Design review of the part built by this model. Coordinates are the model's own, in mm. A direction names the side the tool comes from. Round coordinates to 2 decimals unless told otherwise and drop trailing zeros. Loops run counter-clockwise (first coordinate to the right, second up) from the corner with the lowest first, then second, coordinate; pieces in that order, holes last. Notation, with made-up numbers: (-15.75, 32.25) - (4.25, 32.25) arc R32 ccw to (4.25, 59.25) - close; hole circle Ø3 at (3, 58). An arc over 180 degrees is marked (long way). Use one line per item in the form item = value. Start each with the question number.
(1) Wall thickness on probe 1 along X at (y, z) = (-131, -670); probe 2 along Y at (x, z) = (157, -182); probe 3 along X at (y, z) = (17.5, -85): over which ranges is each line inside the solid? List them lowest first. Write a range as [from, to].
(2) For pin 1 (4 mm diameter, centred on y = -19, z = -359.5, fed in from +X); pin 2 (1.5 mm diameter, centred on x = 870, z = -256, fed in from -Y), all flat-tipped, find the tip position at first contact; note any pin that passes through.
(3) We need section A-A, the plane y = -92. Write out the cut boundary in (x, z).
(4) We need section C-C, the plane y = 26. Write out the cut boundary in (x, z), then the cut area to 3 significant figures.
(5) Machinability: for faces 1 (the cylindrical face through (277.636, 20.28, -249.322)), 2 (the flat face through (913, 11, 0)), 3 (the flat face through (492, 0, -608)), which of the approach directions +Z, -Z, +X, -X, +Y, -Y give a long, thin tool a straight path to every point of the face, cutting with its end or side? Answer none if there is none.
(6) We need section D-D, the plane x = 549. Write out the cut boundary in (y, z), then the cut area to 3 significant figures.
(7) We need section B-B, the plane z = -532. Write out the cut boundary in (x, y).
from build123d import *

# Parameters (mm, degrees)
SKETCH1_W           = 1000
SKETCH1_H           = 1200
BOSS_EXTRUDE1_DEPTH = 40
SKETCH2_W           = 44.100266395
SKETCH2_H           = 1200
SKETCH2_W_2         = 40
BOSS_EXTRUDE2_DEPTH = 140
FILLET1_R           = 70
SKETCH3_R           = 334.802588384
CUT_EXTRUDE2_DEPTH  = 140


with BuildPart() as part:
    # Sketch1 → Boss-Extrude1 (new body)
    with BuildSketch(Plane(origin=(0, 0, 0), x_dir=(1, 0, 0), z_dir=(0, 1, 0))):
        with Locations((500, 600)):
            Rectangle(SKETCH1_W, SKETCH1_H)
    extrude(amount=BOSS_EXTRUDE1_DEPTH)

    # Sketch2 → Boss-Extrude2 (add)
    with BuildSketch(Plane.XZ):
        with Locations((977.949866803, -600)):
            Rectangle(SKETCH2_W, SKETCH2_H)
        with Locations((20, -600)):
            Rectangle(SKETCH2_W_2, SKETCH2_H)
    extrude(amount=BOSS_EXTRUDE2_DEPTH)

    # Fillet1
    fillet1_edges = [part.edges().sort_by_distance(p)[0] for p in [
        (1000, 40, -600),
        (0, 40, -600),
    ]]
    fillet(fillet1_edges, radius=FILLET1_R)

    # Sketch3 → Cut-Extrude2 (cut)
    with BuildSketch(Plane(origin=(0, 40, 0), x_dir=(1, 0, 0), z_dir=(0, 1, 0))):
        with Locations((500, 1200)):
            Circle(SKETCH3_R)
        with BuildLine():
            Line((221.441080201, 0), (780, 0))
            ThreePointArc((780, 0), (725.321357402, 246.103392604), (571.573934725, 445.899197935))
            ThreePointArc((571.573934725, 445.899197935), (500.7205401, 471.613897531), (429.867145476, 445.899197935))
            ThreePointArc((429.867145476, 445.899197935), (276.119722799, 246.103392604), (221.441080201, 0))
        make_face()
    extrude(amount=-CUT_EXTRUDE2_DEPTH, mode=Mode.SUBTRACT)


solid = part.part
Data:
q1.probe_1 = [0, 40], [955.9, 1000]
q1.probe_2 = [0, 40]
q1.probe_3 = [18.58, 227.69], [773.75, 981.42]
q2.pin_1 = 999.42
q2.pin_2 = 0
q3.outline = (0, -1200) - (40, -1200) - (40, 0) - (0, 0) - close; (955.9, -1200) - (1000, -1200) - (1000, 0) - (955.9, 0) - close
q4.outline = (28, -1200) - (165.2, -1200) arc R334.8 cw to (834.8, -1200) - (972, -1200) - (972, 0) - (780, 0) arc R581.18 cw to (571.57, -445.9) arc R110.47 cw to (429.87, -445.9) arc R581.18 cw to (221.44, 0) - (28, 0) - close
q4.area = 762,000 mm^2
q5.face_1 = +Z, +Y, -Y
q5.face_2 = +Z, +X, -X, +Y, -Y
q5.face_3 = +Z, -Z, -Y
q6.outline = (0, -868.8) - (40, -868.8) - (40, -460.51) - (0, -460.51) - close
q6.area = 16,300 mm^2
q7.outline = (0, -140) - (40, -140) - (40, 0) - (955.9, 0) - (955.9, -140) - (1000, -140) - (1000, -30) arc R70 ccw to (930, 40) - (70, 40) arc R70 ccw to (0, -30) - close
